from build123d import *

# Parameters (mm, degrees)
EXTRUDE_2_DEPTH             = 6
HOLE_WIZARD_M41_D           = 4.5
HOLE_WIZARD_M41_CBORE_D     = 8
HOLE_WIZARD_M41_CBORE_DEPTH = 4
SKETCH_13_R                 = 5
SKETCH_13_R_2               = 3.5
CUT_EXTRUDE_1_DEPTH         = 7
FILLET_1_R                  = 5
HOLE_WIZARD_1_4_202_D       = 5.1054
HOLE_WIZARD_3_8_161_D       = 7.9375
HOLE_WIZARD_1_4_203_D       = 5.1054
HOLE_WIZARD_3_8_163_D       = 7.9375


with BuildPart() as part:
    # Эскиз5 → Бобышка-Вытянуть2 (new body)
    with BuildSketch(Plane.XY):
        Polygon((-75, 21.75), (-65, 31.75), (65, 31.75), (75, 21.75), (75, -21.75), (65, -31.75), (-65, -31.75), (-75, -21.75), align=None)
    extrude(amount=EXTRUDE_2_DEPTH)

    # Цековка для винта с внутренним шестигранником M41 (through all)
    with Locations(Plane.XY.offset(6)):
        with Locations((-25, 26.75), (-25, -26.75), (25, -26.75), (25, 26.75)):
            CounterBoreHole(HOLE_WIZARD_M41_D / 2, HOLE_WIZARD_M41_CBORE_D / 2, HOLE_WIZARD_M41_CBORE_DEPTH)

    # Эскиз13 → Вырез-Вытянуть1 (cut, through all)
    with BuildSketch(Plane.XY.offset(6)):
        with Locations((-54.451239655, 7.75)):
            Circle(SKETCH_13_R)
        with Locations((-65.388741386, 16.75)):
            Circle(SKETCH_13_R_2)
        with Locations((-65.388741386, -16.75)):
            Circle(SKETCH_13_R_2)
        with Locations((65.388741386, -16.75)):
            Circle(SKETCH_13_R_2)
        with Locations((54.451239655, 7.75)):
            Circle(SKETCH_13_R)
        with Locations((65.388741386, 16.75)):
            Circle(SKETCH_13_R_2)
        with Locations((0, -16.75)):
            Circle(SKETCH_13_R_2)
        with Locations((-42.5, 0)):
            Circle(SKETCH_13_R_2)
        with Locations((0, 16.75)):
            Circle(SKETCH_13_R)
        with Locations((42.5, 0)):
            Circle(SKETCH_13_R_2)
        with BuildLine():
            Line((-34.207920637, 24.55), (-62.016348651, 24.55))
            ThreePointArc((-62.016348651, 24.55), (-64.116348651, 26.65), (-62.016348651, 28.75))
            Line((-62.016348651, 28.75), (-34.207920637, 28.75))
            ThreePointArc((-34.207920637, 28.75), (-32.107920637, 26.65), (-34.207920637, 24.55))
        make_face()
        with BuildLine():
            Line((34.207920637, 24.55), (62.016348651, 24.55))
            ThreePointArc((62.016348651, 24.55), (64.116348651, 26.65), (62.016348651, 28.75))
            Line((62.016348651, 28.75), (34.207920637, 28.75))
            ThreePointArc((34.207920637, 28.75), (32.107920637, 26.65), (34.207920637, 24.55))
        make_face()
        with BuildLine():
            Line((-34.207920637, -24.55), (-62.016348651, -24.55))
            ThreePointArc((-62.016348651, -24.55), (-64.116348651, -26.65), (-62.016348651, -28.75))
            Line((-62.016348651, -28.75), (-34.207920637, -28.75))
            ThreePointArc((-34.207920637, -28.75), (-32.107920637, -26.65), (-34.207920637, -24.55))
        make_face()
        with BuildLine():
            Line((34.207920637, -24.55), (62.016348651, -24.55))
            ThreePointArc((62.016348651, -24.55), (64.116348651, -26.65), (62.016348651, -28.75))
            Line((62.016348651, -28.75), (34.207920637, -28.75))
            ThreePointArc((34.207920637, -28.75), (32.107920637, -26.65), (34.207920637, -24.55))
        make_face()
        with BuildLine():
            Line((-15, 28.75), (15, 28.75))
            ThreePointArc((15, 28.75), (17.1, 26.65), (15, 24.55))
            Line((15, 24.55), (-15, 24.55))
            ThreePointArc((-15, 24.55), (-17.1, 26.65), (-15, 28.75))
        make_face()
        with BuildLine():
            Line((-15, -28.75), (15, -28.75))
            ThreePointArc((15, -28.75), (17.1, -26.65), (15, -24.55))
            Line((15, -24.55), (-15, -24.55))
            ThreePointArc((-15, -24.55), (-17.1, -26.65), (-15, -28.75))
        make_face()
    extrude(amount=-CUT_EXTRUDE_1_DEPTH, mode=Mode.SUBTRACT)

    # Скругление1
    fillet_1_edges = [part.edges().sort_by_distance(p)[0] for p in [
        (65, 31.75, 3),
        (75, 21.75, 3),
        (75, -21.75, 3),
        (65, -31.75, 3),
        (-65, -31.75, 3),
        (-75, -21.75, 3),
        (-75, 21.75, 3),
        (-65, 31.75, 3),
    ]]
    fillet(fillet_1_edges, radius=FILLET_1_R)

    # Отверстие обработанное метчиком 1/4-202 (through all)
    with Locations(Plane.XY.offset(6)):
        with Locations((-67.5, 0), (-39.060049923, 16.75), (-39.060049923, -16.75), (39.060049923, 16.75), (39.060049923, -16.75), (67.5, 0)):
            Hole(HOLE_WIZARD_1_4_202_D / 2)

    # Отверстие обработанное метчиком 3/8-161 (through all)
    with Locations(Plane.XY.offset(6)):
        with Locations((-54.451239655, -7.75), (54.451239655, -7.75)):
            Hole(HOLE_WIZARD_3_8_161_D / 2)

    # Отверстие обработанное метчиком 1/4-203 (through all)
    with Locations(Plane.XY.offset(6)):
        with Locations((0, 0), (-14.849242405, 7.75), (14.849242405, -7.75)):
            Hole(HOLE_WIZARD_1_4_203_D / 2)

    # Отверстие обработанное метчиком 3/8-163 (through all)
    with Locations(Plane.XY.offset(6)):
        with Locations((-14.849242405, -7.75), (14.849242405, 7.75)):
            Hole(HOLE_WIZARD_3_8_163_D / 2)


solid = part.part
Could you check a few things on this model? Use its own coordinates, in mm. A direction names the side the tool comes from. Give positions to 0.01 mm unless a question says otherwise; leave off trailing zeros. Order: outer loops, then holes, each group sorted by start corner. A loop starts at its lowest first (then second) coordinate and runs counter-clockwise, first axis right, second up.
Item 1: I need wall thicknesses on line 1 (Y direction, x = 10, z = 0.45); line 2 (Y direction, x = 42.5, z = 4); line 3 (X direction, y = -6, z = 3.65). Which ranges of each line are inside material? Lowest first, please.
Item 2: If we section it at D-D, the plane y = 26.75: Count the separate pieces of the cut face and the enclosed holes in it, plus the area to 3 significant figures.
Item 3: If we section it at A-A, the plane y = 7.75: Write out the boundary of the cut face in (x, z).
Item 4: For faces 1 (the face through (-23, 25, 2)), 2 (the face through (48, 28.75, 3)), 3 (the face through (70.05, -26.7, 2.96)), which set-ups out of +Z, -Z, +X, -X, +Y, -Y let a thin tool reach every point of the face, with its end or its side?
Item 5: I'm going to push flat-ended pins straight in: pin 1 (12.5 mm diameter, centred on x = 54.45, y = -7.75, fed in from +Z); pin 2 (6.5 mm diameter, centred on x = -54.45, y = -7.75, fed in from +Z); pin 3 (1.5 mm diameter, centred on y = 22, z = 1.5, fed in from -X); pin 4 (5 mm diameter, centred on x = -25, y = -26.75, fed in from +Z). Where does each tip first touch, or does it pass through?
Item 6: If we section it at C-C, the plane x = 0: Write out the boundary of the cut face in (y, z), plus the area to 3 significant figures.
Item 7: If we mould it in two halves opening along X, with no side actions, what happens to faces 4 (the face through (74.61, 21.62, 3.04)), 5 (the face through (-67.968, -14.385, 3.042)), 6 (the face through (-48, 28.75, 3))? For each: pulls with the +X half, pulls with the -X half, needs draft (parallel to the pull), parting line crosses it, or undercut.
Item 8: If we section it at B-B, the plane x = -25: Write out the boundary of the cut face in (y, z).
Values:
1. line 1: y = -31.75 to -28.75, -24.55 to 24.55, 28.75 to 31.75
1. line 2: y = -31.75 to -28.75, -24.55 to -3.5, 3.5 to 24.55, 28.75 to 31.75
1. line 3: x = -75 to -58.01, -50.89 to -18.41, -11.29 to 12.99, 16.71 to 50.89, 58.01 to 75
2. separate pieces: 6
2. enclosed holes: 0
2. area: 169 mm2
3. outline: (-75, 0) - (-59.45, 0) - (-59.45, 6) - (-75, 6) - close; (-49.45, 0) - (-17.4, 0) - (-17.4, 6) - (-49.45, 6) - close; (-12.3, 0) - (10.88, 0) - (10.88, 6) - (-12.3, 6) - close; (18.82, 0) - (49.45, 0) - (49.45, 6) - (18.82, 6) - close; (59.45, 0) - (75, 0) - (75, 6) - (59.45, 6) - close
4. face 1: +Z
4. face 2: +Z, -Z
4. face 3: +Z, -Z, +X, -Y
5. pin 1: stops at z = 6
5. pin 2: passes through
5. pin 3: stops at x = -74.75
5. pin 4: stops at z = 2
6. outline: (-31.75, 0) - (-28.75, 0) - (-28.75, 6) - (-31.75, 6) - close; (-24.55, 0) - (-20.25, 0) - (-20.25, 6) - (-24.55, 6) - close; (-13.25, 0) - (-2.55, 0) - (-2.55, 6) - (-13.25, 6) - close; (2.55, 0) - (11.75, 0) - (11.75, 6) - (2.55, 6) - close; (21.75, 0) - (24.55, 0) - (24.55, 6) - (21.75, 6) - close; (28.75, 0) - (31.75, 0) - (31.75, 6) - (28.75, 6) - close
6. area: 198 mm2
7. face 4: pulls with the +X half
7. face 5: undercut
7. face 6: undercut
8. outline: (-31.75, 0) - (-29, 0) - (-29, 2) - (-30.75, 2) - (-30.75, 6) - (-31.75, 6) - close; (-24.5, 0) - (24.5, 0) - (24.5, 2) - (22.75, 2) - (22.75, 6) - (-22.75, 6) - (-22.75, 2) - (-24.5, 2) - close; (29, 0) - (31.75, 0) - (31.75, 6) - (30.75, 6) - (30.75, 2) - (29, 2) - close
